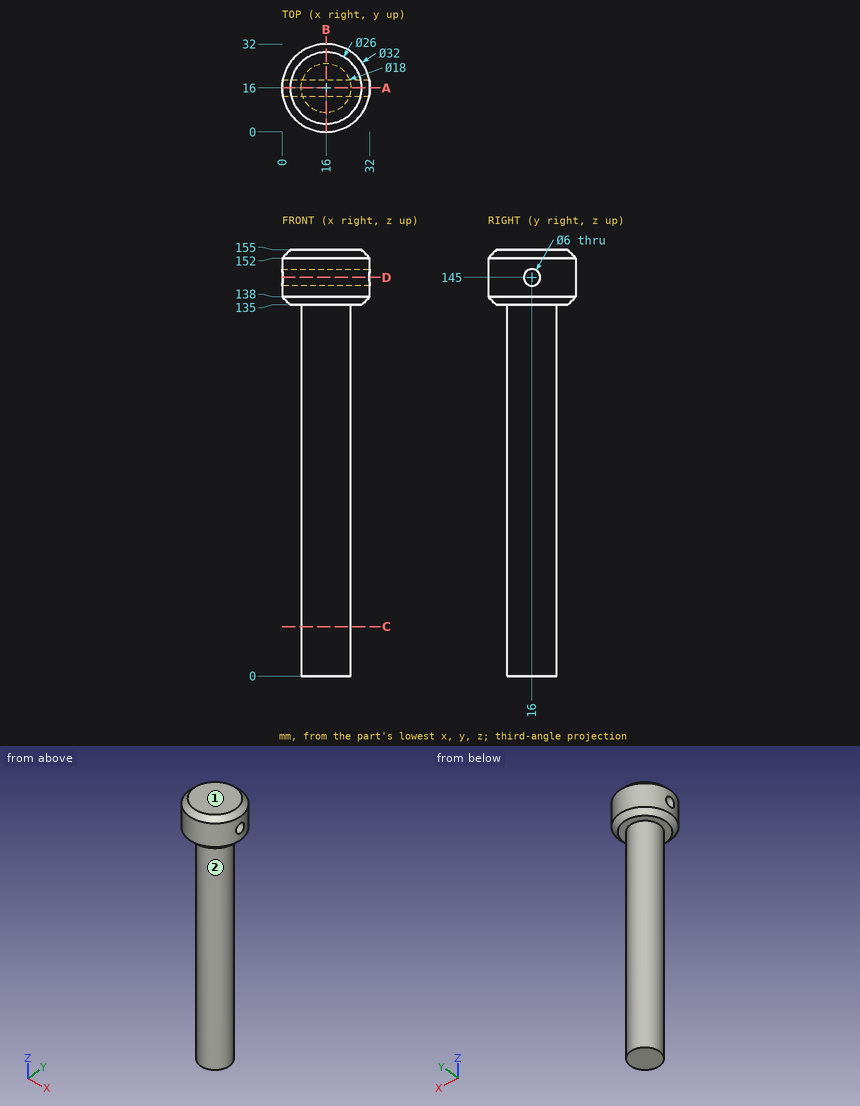
Here's the drawing with two shaded views (mm, measured from the low corner). I have some questions. A direction names the side the tool comes from. Round coordinates to 2 decimals unless told otherwise and drop trailing zeros. Order: outer loops, then holes, each group sorted by start corner. A loop starts at its lowest first (then second) coordinate and runs counter-clockwise, first axis right, second up. Notation, with made-up numbers: (-4, -23.5) -> (0, -23.5) arc R28 ccw to (0, 6.5) -> close; hole circle Ø8 at (36, -32). An arc over 180 degrees is marked (long way). Write each question's results on one line, items separated by ' | '. Start each with the question number.
Item 1: If we section it at A-A, the plane y = 16: Write out the boundary of the cut face in (x, z).
Item 2: If we section it at B-B, the plane x = 16: Write out the boundary of the cut face in (y, z), then the cut area to 3 significant figures.
Item 3: Will these pins go through, and if not, where does the flat tip stop? pin 1 (5 mm diameter, centred on y = 11, z = 74, fed in from -X); pin 2 (4 mm diameter, centred on y = 3.5, z = 60, fed in from -X); pin 3 (10 mm diameter, centred on x = 19, z = 84, fed in from -Y); pin 4 (10 mm diameter, centred on y = 10, z = 85.5, fed in from +X).
Item 4: If we section it at C-C, the plane z = 18: Write out the boundary of the cut face in (x, y).
Item 5: Please list where these lines run through material, in increasing order: L1, parallel to Y at x = 16.5, z = 145; L2, parallel to Y at x = 14, z = 145; L3, parallel to Z at x = 10, y = 26.
Item 6: If we section it at D-D, the plane z = 145: Write out the boundary of the cut face in (x, y).
Item 7: Which directions (+Z, -Z, +X, -X, +Y, -Y) give clear straight access to the entire face, cutting with the end or side of a thin tool? Please do the marked faces 1 and 2.
Results:
1) outline: (0, 138) -> (3, 135) -> (7, 135) -> (7, 0) -> (25, 0) -> (25, 135) -> (29, 135) -> (32, 138) -> (32, 142) -> (0, 142) -> close; (0, 148) -> (32, 148) -> (32, 152) -> (29, 155) -> (3, 155) -> (0, 152) -> close
2) outline: (0, 138) -> (3, 135) -> (7, 135) -> (7, 0) -> (25, 0) -> (25, 135) -> (29, 135) -> (32, 138) -> (32, 152) -> (29, 155) -> (3, 155) -> (0, 152) -> close; hole circle Ø6 at (16, 145) | area: 3,020 mm2
3) pin 1: stops at x = 7.35 | pin 2: passes through | pin 3: stops at y = 7 | pin 4: stops at x = 24.94
4) outline: circle Ø18 at (16, 16)
5) L1: y = 0.01 to 13, 19 to 31.99 | L2: y = 0.13 to 13, 19 to 31.87 | L3: z = 135 to 155
6) outline: (0.28, 13) arc R16 ccw to (31.72, 13) -> close; (0.28, 19) -> (31.72, 19) arc R16 ccw to start
7) face 1: +Z, +X, -X, +Y, -Y | face 2: -Z
